Autodesk Inventor part; units mm, degrees
ref_plane "YZ Plane" through (0, 0, 0) normal (1, 0, 0) x (0, 1, 0)
ref_plane "XZ Plane" through (0, 0, 0) normal (0, 1, 0) x (-1, 0, 0)
ref_plane "XY Plane" through (0, 0, 0) normal (0, 0, 1) x (1, 0, 0)
sketch "Sketch1" plane through (0, 0, 0) normal (0, 1, 0) x (-1, 0, 0)
  circle A0 centre (0, 0) radius 14.2875
  arc A1 (0, -20.6375) -> (0, 20.6375) centre (0, 0) ccw
  line L0 (0, 20.6375) -> (-50.8, 20.6375)
  line L1 (0, -20.6375) -> (-50.8, -20.6375)
  line L2 (-50.8, -20.6375) -> (-50.8, -7.9375)
  line L3 (-50.8, 20.6375) -> (-50.8, 7.9375)
  arc A2 (-50.8, -7.9375) -> (-50.8, 7.9375) centre (-51.136, 0) ccw
  line L4 (-50.8, 14.2875) -> (-38.1, 14.2875) construction
  line L5 (-50.8, -14.2875) -> (-38.1, -14.2875) construction
  circle A3 centre (-38.1, -14.2875) radius 2.5797
  circle A4 centre (-38.1, 14.2875) radius 2.5797
  dimension "d0" = 28.575
  dimension "d1" = 6.35
  dimension "d2" = 50.8
  dimension "d3" = 50.8
  dimension "d4" = 12.7
  dimension "d5" = 12.7
  dimension "d6" = 12.7
  dimension "d7" = 5.1594
  dimension "d8" = 5.1594
extrude "Extrusion1" add sketch "Sketch1" along normal blind 3.175
properties part number "motor connector"
Geometry check sheet. Reference: the model listing, model coordinates, mm. Give positions to 0.01 mm unless a question says otherwise; leave off trailing zeros. Write each loop counter-clockwise with the first axis right and the second up, starting at its lowest first coordinate (ties: lowest second). Pieces come first, ordered by that corner, then holes. Notation, with made-up numbers: M 50,54.25 L 92,54.25 A24 ccw 92,88.25 Z; hole C 11.25,-40 d5. An arc over 180 degrees is marked long. One line per question, with ' | ' between items.
1. Scan lines: line 1 along Z through (x, y) = (38.1, 1.3); line 2 along Z through (x, y) = (0, 1.2); line 3 along X through (y, z) = (2.7, 12.5). Record each from-to range of solid material in increasing order. Write a range as from..to.
Ans:
line 1: -20.64..-16.87, -11.71..11.71, 16.87..20.64 | line 2: -20.64..-14.29, 14.29..20.64 | line 3: -16.42..-6.92, 6.92..36.24, 39.96..50.8
2. Mould release check, pull along X, two halves, no side actions. Record for faces 1 (the face through (24, 0, 0)), 2 (the face through (40.677, 1.565, -14.401)), 3 (the face through (50.8, 2, 14)): released by +X, released by -X, zero draft, split by the parting line, or undercut.
Ans:
face 1: zero draft | face 2: undercut | face 3: released by +X
3. Cross-section at D-D (x = -6). Enter the section's corners in (y, z) (3 decimals), plus the area to 3 significant figures.
Ans:
outline: M 0,-19.746 L 3.175,-19.746 L 3.175,-12.967 L 0,-12.967 Z; M 0,12.967 L 3.175,12.967 L 3.175,19.746 L 0,19.746 Z | area: 43.0 mm2
4. Cross-section at C-C (x = 38.1). Enter the section's corners in (y, z) (1 decimal).
Ans:
outline: M 0,-20.6 L 3.2,-20.6 L 3.2,-16.9 L 0,-16.9 Z; M 0,-11.7 L 3.2,-11.7 L 3.2,11.7 L 0,11.7 Z; M 0,16.9 L 3.2,16.9 L 3.2,20.6 L 0,20.6 Z
5. Gauge pin test, flat ends, axial feed: pin 1 (23 mm diameter, centred on x = 0, z = 0, fed in from +Y); pin 2 (1 mm diameter, centred on y = 2, z = -8, fed in from -X). Record the tip position at first contact, or that the pin passes through.
Ans:
pin 1: through | pin 2: x = -19.23
6. Cross-section at A-A (z = 0). Enter the section's corners in (x, y) (1 decimal).
Ans:
outline: M -20.6,0 L -14.3,0 L -14.3,3.2 L -20.6,3.2 Z; M 14.3,0 L 43.2,0 L 43.2,3.2 L 14.3,3.2 Z
7. Cross-section at B-B (y = 1.7). Enter the section's corners in (x, z) (1 decimal), plus the area to 3 significant figures.
Ans:
outline: M 0,-20.6 L 50.8,-20.6 L 50.8,-7.9 A7.9 cw 50.8,7.9 L 50.8,20.6 L 0,20.6 A20.6 ccw Z; hole C 0,0 d28.6; hole C 38.1,-14.3 d5.2; hole C 38.1,14.3 d5.2 | area: 1,990 mm2
